```python
from build123d import *

# Parameters (mm, degrees)
SKETCH1_W           = 135
SKETCH1_H           = 72.5
BOSS_EXTRUDE1_DEPTH = 12
SKETCH2_W           = 131
SKETCH2_H           = 68.5
BOSS_EXTRUDE2_DEPTH = 4
SKETCH4_W           = 128.6
SKETCH4_H           = 66.1
CUT_EXTRUDE1_DEPTH  = 4
SKETCH5_W           = 128.6
SKETCH5_H           = 66.1
CUT_EXTRUDE2_DEPTH  = 8
SKETCH6_W           = 1.5
SKETCH6_H           = 66.1
CUT_EXTRUDE3_DEPTH  = 10


with BuildPart() as part:
    # Sketch1 → Boss-Extrude1 (new body)
    with BuildSketch(Plane.XY):
        with Locations((62.683098592, -32.088028169)):
            Rectangle(SKETCH1_W, SKETCH1_H)
    extrude(amount=BOSS_EXTRUDE1_DEPTH)

    # Sketch2 → Boss-Extrude2 (add)
    with BuildSketch(Plane.XY.offset(12)):
        with Locations((62.683098592, -32.088028169)):
            Rectangle(SKETCH2_W, SKETCH2_H)
    extrude(amount=BOSS_EXTRUDE2_DEPTH)

    # Sketch4 → Cut-Extrude1 (cut)
    with BuildSketch(Plane.XY.offset(16)):
        with Locations((62.683098592, -32.088028169)):
            Rectangle(SKETCH4_W, SKETCH4_H)
    extrude(amount=-CUT_EXTRUDE1_DEPTH, mode=Mode.SUBTRACT)

    # Sketch5 → Cut-Extrude2 (cut)
    with BuildSketch(Plane.XY.offset(12)):
        with Locations((62.683098592, -32.088028169)):
            Rectangle(SKETCH5_W, SKETCH5_H)
    extrude(amount=-CUT_EXTRUDE2_DEPTH, mode=Mode.SUBTRACT)

    # Sketch6 → Cut-Extrude3 (cut)
    with BuildSketch(Plane(origin=(128.183098592, 0, 0), x_dir=(0, 0, -1), z_dir=(1, 0, 0))):
        with Locations((-15.25, -32.088028169)):
            Rectangle(SKETCH6_W, SKETCH6_H)
    extrude(amount=-CUT_EXTRUDE3_DEPTH, mode=Mode.SUBTRACT)


solid = part.part
```
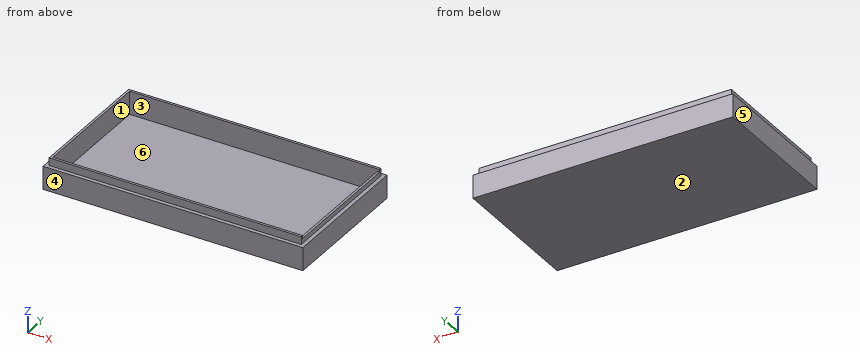
Can you work these out from the model? Positions are in its coordinate system, mm. Face numbers are marked on the shaded views. A direction names the side the tool comes from. Coordinates: 2 decimals unless noted, no trailing zeros. Order: outer loops, then holes, each group sorted by start corner. A loop starts at its lowest first (then second) coordinate and runs counter-clockwise, first axis right, second up. Notation, with made-up numbers: (-20, -20) - (38, -20) arc R17 cw to (38, -12) - close; hole circle Ø8 at (26, 47.25). An arc over 180 degrees is marked (long way). Answer in a Markdown table with one row per item.
1. Suppose I cut it at C-C (x = 103.5). Please give me the cut outline in (y, z), and give its area (3 significant figures).
Reply:
| item | result |
|---|---|
| outline | (-68.34, 0) - (4.16, 0) - (4.16, 12) - (2.16, 12) - (2.16, 16) - (0.96, 16) - (0.96, 4) - (-65.14, 4) - (-65.14, 16) - (-66.34, 16) - (-66.34, 12) - (-68.34, 12) - close |
| area | 351 mm^2 |
2. If we mould it in two halves opening along Y, with no side actions, what happens to the marked faces 1, 2, 3 and 4? For each: pulls with the +Y half, pulls with the -Y half, needs draft (parallel to the pull), parting line crosses it, or undercut.
Reply:
| item | result |
|---|---|
| face 1 | undercut |
| face 2 | needs draft |
| face 3 | undercut |
| face 4 | pulls with the -Y half |
3. Suppose I cut it at A-A (z = 9). Please give me the cut outline in (x, y).
Reply:
| item | result |
|---|---|
| outline | (-4.82, -68.34) - (130.18, -68.34) - (130.18, 4.16) - (-4.82, 4.16) - close; hole (-1.62, -65.14) - (126.98, -65.14) - (126.98, 0.96) - (-1.62, 0.96) - close |
4. Suppose I cut it at B-B (y = -51). Please give me the cut outline in (x, z).
Reply:
| item | result |
|---|---|
| outline | (-4.82, 0) - (130.18, 0) - (130.18, 12) - (128.18, 12) - (128.18, 14.5) - (126.98, 14.5) - (126.98, 4) - (-1.62, 4) - (-1.62, 16) - (-2.82, 16) - (-2.82, 12) - (-4.82, 12) - close |
5. For the marked faces 5 and 6, which set-ups out of +Z, -Z, +X, -X, +Y, -Y let a thin tool reach every point of the face, with its end or its side?
Reply:
| item | result |
|---|---|
| face 5 | +Z, -Z, -X, +Y, -Y |
| face 6 | +Z |
6. If I drill on line 1 along Y through (x, z) = (82.5, 6.75); line 2 along X through (y, z) = (-17, 8); line 3 along X through (y, z) = (-56.5, 13.5), over which ranges is the centre line in solid material (lowest first)?
Reply:
| item | result |
|---|---|
| line 1 | y = -68.34 to -65.14, 0.96 to 4.16 |
| line 2 | x = -4.82 to -1.62, 126.98 to 130.18 |
| line 3 | x = -2.82 to -1.62, 126.98 to 128.18 |
7. For pin 1 (2 mm diameter, centred on x = 84.5, y = -61, fed in from +Z); pin 2 (1.5 mm diameter, centred on y = -47.5, z = 14, fed in from +X); pin 3 (1 mm diameter, centred on x = 127.5, y = -31, fed in from +Z), each with a flat end and sliding along its axis, tell me the tip position at first contact or that it passes through.
Reply:
| item | result |
|---|---|
| pin 1 | stops at z = 4 |
| pin 2 | stops at x = 128.18 |
| pin 3 | stops at z = 14.5 |
